```python
from build123d import *

# Parameters (mm, degrees)
SKETCH1_W           = 20
SKETCH1_H           = 10
BOSS_EXTRUDE1_DEPTH = 3
SKETCH2_W           = 9.8
SKETCH2_H           = 8.5
SKETCH2_W_2         = 5.8
SKETCH2_H_2         = 4.5
BOSS_EXTRUDE2_DEPTH = 3
BOSS_EXTRUDE3_DEPTH = 1


with BuildPart() as part:
    # Sketch1 → Boss-Extrude1 (new body)
    with BuildSketch(Plane(origin=(0, 0, 0), x_dir=(1, 0, 0), z_dir=(0, 1, 0))):
        Rectangle(SKETCH1_W, SKETCH1_H)
    extrude(amount=BOSS_EXTRUDE1_DEPTH)

    # Sketch2 → Boss-Extrude2 (add)
    with BuildSketch(Plane.XZ):
        Rectangle(SKETCH2_W, SKETCH2_H)
        Rectangle(SKETCH2_W_2, SKETCH2_H_2, mode=Mode.SUBTRACT)
    extrude(amount=BOSS_EXTRUDE2_DEPTH)

    # Sketch3 → Boss-Extrude3 (add)
    with BuildSketch(Plane(origin=(0, 3, 0), x_dir=(1, 0, 0), z_dir=(0, 1, 0))):
        with BuildLine():
            add(Edge.make_bspline(
                [(-3.007246377, -1.541055254), (-3.009361723, -1.616266832), (-3.01346546, -1.762176027), (-3.049571221, -1.974490768), (-3.109784234, -2.171698983), (-3.192526507, -2.355150602), (-3.298968583, -2.521513857), (-3.420549524, -2.676791882), (-3.565727351, -2.813375097), (-3.726560117, -2.937740496), (-3.905559946, -3.047190671), (-4.103184871, -3.139302997), (-4.316725708, -3.21887973), (-4.54677574, -3.283042654), (-4.79127798, -3.332920655), (-5.049025563, -3.367185197), (-5.318723514, -3.390311379), (-5.502591678, -3.39288864), (-5.596354167, -3.394202899)],
                knots=[0, 0, 0, 0, 1.005643061, 1.95093061, 2.870738502, 3.757832008, 4.633806625, 5.507195241, 6.389247641, 7.292512577, 8.223494331, 9.189475669, 10.205094408, 11.269007441, 12.381228937, 13.540657028, 14.745872513, 16, 16, 16, 16], degree=3))
            add(Edge.make_bspline(
                [(-5.596354167, -3.394202899), (-5.682718588, -3.393235229), (-5.855033921, -3.391304522), (-6.111280949, -3.379468444), (-6.361973178, -3.359915664), (-6.603364511, -3.33640358), (-6.833625513, -3.310266833), (-7.049705719, -3.280039115), (-7.248879542, -3.244891381), (-7.374986232, -3.218371914), (-7.434782609, -3.205797101)],
                knots=[0, 0, 0, 0, 1.119729043, 2.234096861, 3.324996266, 4.379512959, 5.378439906, 6.329323539, 7.207810484, 8, 8, 8, 8], degree=3))
            Line((-7.434782609, -3.205797101), (-7.434782609, -2.357971014))
            add(Edge.make_bspline(
                [(-7.434782609, -2.357971014), (-7.370762942, -2.379906097), (-7.239954637, -2.424724996), (-7.034769621, -2.477293495), (-6.819537264, -2.526663443), (-6.592212353, -2.567908961), (-6.350580188, -2.600371202), (-6.09371887, -2.623201503), (-5.82076552, -2.638661997), (-5.633665552, -2.639928566), (-5.537477355, -2.64057971)],
                knots=[0, 0, 0, 0, 0.842364813, 1.72116351, 2.635659137, 3.591954833, 4.596841017, 5.670471508, 6.802388115, 8, 8, 8, 8], degree=3))
            add(Edge.make_bspline(
                [(-5.537477355, -2.64057971), (-5.468755519, -2.639872283), (-5.336572064, -2.638511576), (-5.146102436, -2.624285716), (-4.971197978, -2.605738792), (-4.812235473, -2.573524326), (-4.66761954, -2.536445211), (-4.53690496, -2.489260746), (-4.420297965, -2.43310849), (-4.315764365, -2.370159285), (-4.226176786, -2.297427118), (-4.14763217, -2.219043718), (-4.08459987, -2.131603251), (-4.033398257, -2.037180835), (-3.995547608, -1.93545715), (-3.969262703, -1.826700795), (-3.952727851, -1.711319689), (-3.950446508, -1.631881026), (-3.949275362, -1.591100543)],
                knots=[0, 0, 0, 0, 1.523194236, 2.929797672, 4.233142745, 5.41923506, 6.522104548, 7.540643951, 8.494207191, 9.387815665, 10.238903194, 11.04655015, 11.840679357, 12.619387111, 13.4214478, 14.239285369, 15.096122854, 16, 16, 16, 16], degree=3))
            add(Edge.make_bspline(
                [(-3.949275362, -1.591100543), (-3.950736926, -1.548727509), (-3.953592513, -1.465939512), (-3.982760391, -1.347167725), (-4.028364162, -1.237025632), (-4.095221609, -1.138795344), (-4.173790678, -1.046499637), (-4.266091432, -0.961927422), (-4.367978541, -0.880147855), (-4.522576355, -0.777306411), (-4.738901588, -0.6564636), (-5.027071288, -0.535618888), (-5.332657608, -0.414283489), (-5.646271299, -0.28773006), (-5.959805031, -0.153393094), (-6.267393971, -0.011077429), (-6.555877209, 0.152188183), (-6.773110218, 0.314191425), (-6.924884877, 0.460070087), (-7.028139342, 0.576873874), (-7.116736104, 0.704422635), (-7.19857963, 0.83820536), (-7.26261074, 0.986049766), (-7.307035659, 1.146566576), (-7.336517595, 1.31977591), (-7.339194196, 1.439453928), (-7.34057971, 1.501403986)],
                knots=[0, 0, 0, 0, 0.619815692, 1.2109895, 1.781199776, 2.357496674, 2.943929778, 3.554333405, 4.188738872, 4.856760597, 6.272963823, 7.811824644, 9.431291666, 11.092170587, 12.76691914, 14.429617761, 16.056218893, 17.616396577, 18.384212937, 19.138341755, 19.896401647, 20.65718422, 21.4332038, 22.247956952, 23.09307348, 24, 24, 24, 24], degree=3))
            add(Edge.make_bspline(
                [(-7.34057971, 1.501403986), (-7.338890921, 1.55695311), (-7.335509193, 1.668187842), (-7.30757402, 1.834398802), (-7.263639098, 1.99915748), (-7.201785927, 2.161864622), (-7.120766105, 2.318754545), (-7.022162869, 2.469164015), (-6.90104822, 2.607647577), (-6.762169614, 2.738226423), (-6.601498999, 2.857697029), (-6.421044497, 2.966681175), (-6.217870333, 3.06021036), (-5.995865777, 3.145085669), (-5.75055523, 3.212458991), (-5.483154955, 3.260726864), (-5.193612621, 3.28796892), (-4.993414416, 3.292077257), (-4.889832428, 3.294202899)],
                knots=[0, 0, 0, 0, 0.784067079, 1.570060577, 2.373452904, 3.189297991, 4.022898002, 4.862695015, 5.722463422, 6.614650011, 7.550049647, 8.544652583, 9.586108202, 10.704431291, 11.897970904, 13.172772987, 14.537200697, 16, 16, 16, 16], degree=3))
            add(Edge.make_bspline(
                [(-4.889832428, 3.294202899), (-4.831915002, 3.293827656), (-4.71154814, 3.293047807), (-4.526083854, 3.279715221), (-4.332642127, 3.262900288), (-4.135942453, 3.23881275), (-3.939571378, 3.211313867), (-3.746785439, 3.17889299), (-3.561719244, 3.144290109), (-3.441899158, 3.118329271), (-3.384057971, 3.105797101)],
                knots=[0, 0, 0, 0, 0.91416123, 1.89985515, 2.934260182, 3.979599391, 5.027947684, 6.064525625, 7.065681407, 8, 8, 8, 8], degree=3))
            Line((-3.384057971, 3.105797101), (-3.384057971, 2.352173913))
            add(Edge.make_bspline(
                [(-3.384057971, 2.352173913), (-3.512802353, 2.380728564), (-3.769014174, 2.437554648), (-4.154613263, 2.494241446), (-4.53329374, 2.533940296), (-4.78326578, 2.538393033), (-4.906023551, 2.54057971)],
                knots=[0, 0, 0, 0, 1.029411825, 2.048613503, 3.041701399, 4, 4, 4, 4], degree=3))
            add(Edge.make_bspline(
                [(-4.906023551, 2.54057971), (-4.96785961, 2.539634528), (-5.087722119, 2.537802395), (-5.261250093, 2.526537867), (-5.421923855, 2.50591041), (-5.569906649, 2.478011851), (-5.705607433, 2.443486967), (-5.828608574, 2.399624608), (-5.938232428, 2.346084815), (-6.036323458, 2.285929472), (-6.121441499, 2.217830494), (-6.196267253, 2.145534626), (-6.25873862, 2.066920743), (-6.309166265, 1.982002857), (-6.348629922, 1.891910001), (-6.379278296, 1.797018907), (-6.39483351, 1.695718813), (-6.39729289, 1.626561307), (-6.398550725, 1.591191123)],
                knots=[0, 0, 0, 0, 1.491437277, 2.890989782, 4.191431573, 5.395946596, 6.521058188, 7.565423013, 8.539223212, 9.458660202, 10.334655275, 11.163081303, 11.963306063, 12.748694206, 13.538083787, 14.331542868, 15.146677777, 16, 16, 16, 16], degree=3))
            add(Edge.make_bspline(
                [(-6.398550725, 1.591191123), (-6.397090804, 1.54882223), (-6.394238428, 1.466042324), (-6.364939026, 1.346770736), (-6.319091437, 1.236318933), (-6.254990308, 1.135022601), (-6.173334725, 1.044741827), (-6.083461638, 0.956922737), (-5.981213723, 0.874535374), (-5.826918921, 0.769047924), (-5.608685055, 0.648834692), (-5.321927803, 0.522708732), (-5.01464681, 0.404830914), (-4.701773525, 0.277036411), (-4.387114081, 0.144096978), (-4.130666417, 0.020425333), (-3.931637116, -0.085736683), (-3.792159425, -0.174732598), (-3.659724913, -0.268594319), (-3.537951241, -0.372291237), (-3.423674946, -0.481967024), (-3.321521117, -0.602520833), (-3.230395949, -0.731327418), (-3.151822879, -0.869682551), (-3.084616777, -1.017867369), (-3.040791314, -1.18089857), (-3.011296839, -1.356483959), (-3.008627503, -1.478120166), (-3.007246377, -1.541055254)],
                knots=[0, 0, 0, 0, 0.667485538, 1.304126353, 1.925325377, 2.548259058, 3.18485279, 3.841928735, 4.529978862, 5.253739616, 6.789399884, 8.452896455, 10.194043647, 11.982660287, 13.786213269, 15.583473082, 16.473910229, 17.343881083, 18.192645259, 19.033319022, 19.865571682, 20.689426309, 21.522902605, 22.351690537, 23.197589349, 24.082454772, 25.007853999, 26, 26, 26, 26], degree=3))
        make_face()
        Polygon((2.268115942, -3.3), (-1.405797101, -3.3), (-1.405797101, 3.2), (2.268115942, 3.2), (2.268115942, 2.446376812), (-0.463768116, 2.446376812), (-0.463768116, 0.468115942), (2.159193841, 0.468115942), (2.159193841, -0.285507246), (-0.463768116, -0.285507246), (-0.463768116, -2.546376812), (2.268115942, -2.546376812), align=None)
        Polygon((8.014492754, -3.3), (4.246376812, -3.3), (4.246376812, 3.2), (5.188405797, 3.2), (5.188405797, -2.546376812), (8.014492754, -2.546376812), align=None)
    extrude(amount=BOSS_EXTRUDE3_DEPTH)


solid = part.part
```
Design review of the part built by this model. Coordinates are the model's own, in mm. A direction names the side the tool comes from. Give positions to 0.01 mm unless a question says otherwise; leave off trailing zeros. Order: outer loops, then holes, each group sorted by start corner. A loop starts at its lowest first (then second) coordinate and runs counter-clockwise, first axis right, second up. Notation, with made-up numbers: (-11, 13.5) -> (14, 13.5) arc R13 cw to (14, 36.5) -> close; hole circle Ø5 at (12, 20.5). An arc over 180 degrees is marked (long way). Write item = value, one per line. Start each with the question number.
(1) We need section B-B on x = 3.25. Write out the cut boundary in (y, z), plus the area to 3 significant figures.
(2) We need section D-D on x = 0.5. Write out the cut boundary in (y, z), plus the area to 3 significant figures.
(3) For pin 1 (0.8 mm diameter, centred on y = 3.5, z = -3, fed in from +X); pin 2 (3 mm diameter, centred on y = -0.5, z = 3, fed in from -X); pin 3 (2 mm diameter, centred on y = -2, z = 1.5, fed in from +X); pin 4 (0.9 mm diameter, centred on x = 1, y = -1, fed in from -Z), all flat-tipped, find the tip position at first contact; note any pin that passes through.
(4) For faces 4 (the face through (0, -1, -4.25)), 5 (the face through (-2.9, -1, 0)), 6 (the face through (0.9, 3.5, 2.546)), 7 (the face through (4.246, 3.5, 0.1)), list the 3-axis set-ups (+Z, -Z, +X, -X, +Y, -Y) from which the entire face can be reached by the end or side of a thin tool; tool diameter is ignored.
(5) We need section A-A on y = -1. Write out the cut boundary in (x, z).
(6) Mouldability with a two-part tool opening along Z and no side actions: class faces 1 (the face through (4.7, 3.5, -3.2)), 2 (the face through (2.9, -1, 0)), 3 (the face through (0, 1, 5)) as +Z half, -Z half, draft (parallel to the pull), parting line (faces both ways), or undercut.
(7) We need section C-C on z = 4. Write out the cut boundary in (x, y), plus the area to 3 significant figures.
(8) To check wall thickness, follow line 1 along Z through (x, y) = (0, 3.5); line 2 along Z through (x, y) = (1.5, -2.5); line 3 along X through (y, z) = (-1, -1). State the ranges of each line that lie inside material, in increasing order.
Numbers:
q1.outline = (-3, -4.25) -> (0, -4.25) -> (0, -5) -> (3, -5) -> (3, 5) -> (0, 5) -> (0, 4.25) -> (-3, 4.25) -> close
q1.area = 55.5 mm^2
q2.outline = (-3, -4.25) -> (0, -4.25) -> (0, -5) -> (3, -5) -> (3, -3.2) -> (4, -3.2) -> (4, -2.45) -> (3, -2.45) -> (3, -0.47) -> (4, -0.47) -> (4, 0.29) -> (3, 0.29) -> (3, 2.55) -> (4, 2.55) -> (4, 3.3) -> (3, 3.3) -> (3, 5) -> (0, 5) -> (0, 4.25) -> (-3, 4.25) -> (-3, 2.25) -> (0, 2.25) -> (0, -2.25) -> (-3, -2.25) -> close
q2.area = 44.3 mm^2
q3.pin_1 = 5.19
q3.pin_2 = -10
q3.pin_3 = 4.9
q3.pin_4 = -4.25
q4.face_4 = -Z, +X, -X, -Y
q4.face_5 = -Y
q4.face_6 = +Y
q4.face_7 = +Z, -Z, +Y
q5.outline = (-4.9, -4.25) -> (4.9, -4.25) -> (4.9, 4.25) -> (-4.9, 4.25) -> close; hole (-2.9, -2.25) -> (2.9, -2.25) -> (2.9, 2.25) -> (-2.9, 2.25) -> close
q6.face_1 = -Z half
q6.face_2 = undercut
q6.face_3 = +Z half
q7.outline = (-10, 0) -> (-4.9, 0) -> (-4.9, -3) -> (4.9, -3) -> (4.9, 0) -> (10, 0) -> (10, 3) -> (-10, 3) -> close
q7.area = 89.4 mm^2
q8.line_1 = -3.2 to -2.45, -0.47 to 0.29, 2.55 to 3.3
q8.line_2 = -4.25 to -2.25, 2.25 to 4.25
q8.line_3 = -4.9 to -2.9, 2.9 to 4.9
